Geometry check sheet. Reference: the model listing, model coordinates, mm. Face numbers are marked on the shaded views. A direction names the side the tool comes from. Give positions to 0.01 mm unless a question says otherwise; leave off trailing zeros. Write each loop counter-clockwise with the first axis right and the second up, starting at its lowest first coordinate (ties: lowest second). Pieces come first, ordered by that corner, then holes. Notation, with made-up numbers: (62, 85.25) - (118, 85.25) arc R34 ccw to (118, 120.25) - close; hole circle Ø11 at (65.25, 77). An arc over 180 degrees is marked (long way). One line per question, with ' | ' between items. Start each with the question number.
Q1. Release check for a two-part mould opening along Z. For the marked faces 1, 2 and 3 record: +Z half, -Z half, draft (parallel to the pull), parting line (faces both ways), or undercut.
Q2. Section check B-B on z = 18. Record the boundary of the cut face in (x, y) (3 decimals), and give its area (3 significant figures).
Q3. Section check A-A on x = -17. Record the boundary of the cut face in (y, z).
Q4. Set-up check for the marked faces 4 and 5: record each of +Z, -Z, +X, -X, +Y, -Y from which the full face is reachable in a straight line by a thin tool's end or side.
Q5. Section check C-C on x = -27.5. Record the boundary of the cut face in (y, z).
Q6. Section check D-D on z = 45. Record the boundary of the cut face in (x, y) (3 decimals), and give its area (3 significant figures).
Q7. Gauge pin test, flat ends, axial feed: P1, Ø1.5, axis at x = 8.5, z = 103.5, coming from the +Y side; P2, Ø6, axis at x = 17, y = 7.5, coming from the +Z side; P3, Ø4, axis at x = 6, z = 46, coming from the +Y side; P4, Ø8, axis at x = 4, z = 28, coming from the +Y side. Record the tip position at first contact, or that the pin passes through.
Q8. Thickness scan on L1, parallel to Y at x = -17, z = 104.05; L2, parallel to Z at x = 15, y = -4; L3, parallel to Y at x = 0.5, z = 99. Record the ranges inside material, lowest first. Write a range as [from, to].
Autodesk Fusion 360 part; units mm, degrees
sketch "Sketch1" plane through (0, 0, 0) normal (0, 0, 1) x (1, 0, 0)
  circle A0 centre (0, 0) radius 7
  circle A1 centre (0, 0) radius 12.5
  dimension "d1" = 25
  dimension "d2" = 14
extrude "Extrude1" add sketch "Sketch1" along normal blind 15 contours A0 | A1
sketch "Sketch2" plane through (0, 0, 15) normal (0, 0, 1) x (1, 0, 0)
  circle A0 centre (0, 0) radius 12.5
  circle A1 centre (0, 0) radius 6.375
  dimension "d5" = 12.75
loft "Loft1" cut profiles "Sketch1", "Sketch2" section 1 contours A0 section 2 contours A1
extrude "Extrude2" add 1 faces at (10.4118, -0.621, 15) along direction (0, 0, 1) blind 92
sketch "Sketch17" plane through (0, 0, 107) normal (0, 0, 1) x (1, 0, 0)
  circle A0 centre (-17, -7.5) radius 2.25
  circle A1 centre (17, -7.5) radius 2.25
  circle A2 centre (0, 0) radius 6.375
  circle A3 centre (0, 0) radius 12.5
  line L0 (-22.5, 13) -> (22.5, 13)
  line L1 (22.5, 13) -> (22.5, -13)
  line L2 (22.5, -13) -> (-22.5, -13)
  line L3 (-22.5, -13) -> (-22.5, 13)
  line L4 (0, 0) -> (-22.5, 0) construction
  line L5 (0, 0) -> (22.5, 0) construction
  circle A4 centre (-17, 7.5) radius 2.25
  circle A5 centre (17, 7.5) radius 2.25
  point P0 (-12.5, 0)
  point P1 (12.5, 0)
  dimension "d112" = 4.5
  dimension "d113" = 4.5
  dimension "d147" = 10
  dimension "d148" = 10
  dimension "d149" = 7.5
  dimension "d150" = 13
  dimension "d151" = 17
  dimension "d152" = 17
  dimension "d153" = 7.5
  dimension "d154" = 17
  dimension "d155" = 7.5
  dimension "d156" = 4.5
  dimension "d157" = 4.5
  dimension "d158" = 17
  dimension "d159" = 7.5
extrude "Extrude15" add sketch "Sketch17" against normal blind 5 contours A3 | L0 L1 L2 L3
sketch "Sketch18" plane through (0, 0, 0) normal (0, 0, -1) x (-1, 0, 0)
  circle A0 centre (-17, -7.5) radius 2.25
  circle A1 centre (17, -7.5) radius 2.25
  line L0 (-34.9564, 15) -> (34.9564, 15)
  line L1 (34.9564, 15) -> (34.9564, -15)
  line L2 (34.9564, -15) -> (-34.9564, -15)
  line L3 (-34.9564, -15) -> (-34.9564, 15)
  circle A2 centre (-27.4564, -7.5) radius 2.25
  circle A3 centre (0, 0) radius 7
  circle A4 centre (0, 0) radius 12.5
  line L4 (-22.5, -13) -> (22.5, -13)
  line L5 (22.5, -13) -> (22.5, 13)
  line L6 (22.5, 13) -> (-22.5, 13)
  line L7 (-22.5, 13) -> (-22.5, -13)
  circle A5 centre (0, 0) radius 12.5
  circle A6 centre (-17, 7.5) radius 2.25
  circle A7 centre (17, 7.5) radius 2.25
  circle A8 centre (-27.4564, 7.5) radius 2.25
  circle A9 centre (27.4564, 7.5) radius 2.25
  point P0 (0, -15)
  dimension "d122" = 4.5
  dimension "d124" = 7.5
  dimension "d125" = 7.5
  dimension "d160" = 34.9564
  dimension "d161" = 15
  dimension "d162" = 34.9564
  dimension "d163" = 15
  dimension "d164" = 7.5
  dimension "d165" = 7.5
  dimension "d166" = 4.5
  dimension "d167" = 7.5
  dimension "d168" = 7.5
  dimension "d169" = 4.5
extrude "Extrude16" add sketch "Sketch18" against normal blind 3 contours A0 | A1 | L0 L1 L2 L3 | L4 L5 L6 L7 | A6 | A7
ref_plane "WorkPlane5" through (0, -7, 0) normal (0, 1, 0) x (0, 0, 1)
sketch "Sketch19" plane through (0, -7, 0) normal (0, 1, 0) x (1, 0, 0)
  line L0 (6.375, -15) -> (-6.375, -15)
  line L1 (0, -15) -> (0, -107) construction
  circle A0 centre (0, -18) radius 1.7
  circle A1 centre (0, -18) radius 2.7
  line L2 (6.375, -107) -> (-6.375, -107)
  dimension "d131" = 3.4
  dimension "d132" = 5.4
  dimension "d139" = 3
extrude "Extrude17" add sketch "Sketch19" against normal blind 8
extrude "Extrude18" cut sketch "Sketch19" along normal blind 2 and the other way blind 8 contours A0
ref_plane "WorkPlane7" through (0, 7, 0) normal (0, 1, 0) x (0, 0, 1)
sketch "Sketch22" plane through (0, 7, 0) normal (0, 1, 0) x (1, 0, 0)
  circle A0 centre (0, -18) radius 1.7
  circle A1 centre (0, -18) radius 2.7
  point P0 (0, -18)
  dimension "d171" = 3.4
  dimension "d172" = 5.4
extrude "Extrude21" add sketch "Sketch22" along normal blind 8
extrude "Extrude22" cut sketch "Sketch22" along normal blind 8 and the other way blind 2 contours A0
sketch "Sketch23" plane through (0, 0, 0) normal (0, 0, -1) x (-1, 0, 0)
  line L0 (-34.9564, -15) -> (34.9564, -15)
  line L1 (34.9564, -15) -> (34.9564, 15)
  line L2 (34.9564, 15) -> (-34.9564, 15)
  line L3 (-34.9564, 15) -> (-34.9564, -15)
  circle A0 centre (-27.4564, 7.5) radius 2.25
  circle A1 centre (-27.4564, -7.5) radius 2.25
  circle A2 centre (27.4564, 7.5) radius 2.25
  circle A3 centre (0, 0) radius 7
  line L4 (34.9564, -15) -> (30.1724, -15)
  line L5 (34.9564, -9.125) -> (34.9564, -15)
  arc A4 (34.9564, -9.125) -> (30.1724, -15) centre (36.8966, -15.5902) ccw
  dimension "d181" = 4.784
  dimension "d182" = 5.875
  dimension "d183" = 6.75
extrude "Extrude23" cut sketch "Sketch23" against normal up to surface (3 mm away) contours L0 L1 L4 L5 A4
equation "d113 = d112"
equation "d116 = d110 / 2"
equation "d125 = d124"
equation "d130 = -d2 / 2"
equation "d132 = d131 + 2 mm"
equation "d148 = d147"
equation "d152 = d151"
equation "d153 = d149"
equation "d154 = d151"
equation "d155 = d149"
equation "d156 = d112"
equation "d157 = d112"
equation "d158 = d151"
equation "d159 = d149"
equation "d162 = d160"
equation "d163 = d161"
equation "d164 = d124"
equation "d165 = d124"
equation "d166 = d122"
equation "d167 = d124"
equation "d168 = d124"
equation "d169 = d122"
equation "d170 = ( d2 / 2 mm ) * 1 mm"
equation "d172 = d171 + 2 mm"
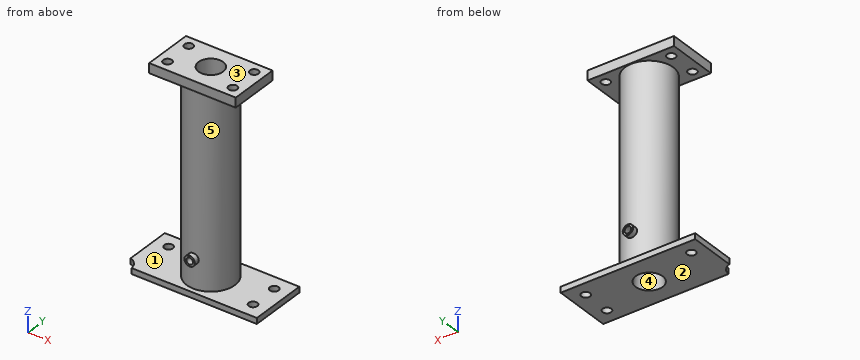
Working result:
1) face 1: undercut | face 2: -Z half | face 3: +Z half
2) outline: (-2.7, -15) - (-1.7, -15) - (-1.7, -6.144) arc R6.375 cw to (-1.7, 6.144) - (-1.7, 15) - (-2.7, 15) - (-2.7, 12.205) arc R12.5 ccw to (-2.7, -12.205) - close; (1.7, -15) - (2.7, -15) - (2.7, -12.205) arc R12.5 ccw to (2.7, 12.205) - (2.7, 15) - (1.7, 15) - (1.7, 6.144) arc R6.375 cw to (1.7, -6.144) - close | area: 332 mm2
3) outline: (-15, 0) - (15, 0) - (15, 3) - (-15, 3) - close; (-13, 102) - (-9.75, 102) - (-9.75, 107) - (-13, 107) - close; (-5.25, 102) - (5.25, 102) - (5.25, 107) - (-5.25, 107) - close; (9.75, 102) - (13, 102) - (13, 107) - (9.75, 107) - close
4) face 4: -Z | face 5: none
5) outline: (-15, 0) - (5.25, 0) - (5.25, 3) - (-15, 3) - close; (9.75, 0) - (15, 0) - (15, 3) - (9.75, 3) - close
6) outline: circle Ø25 at (0, 0); hole circle Ø12.75 at (0, 0) | area: 363 mm2
7) P1: stops at y = 13 | P2: stops at z = 107 | P3: stops at y = 11.84 | P4: stops at y = 12.5
8) L1: y = [-13, -9.75], [-5.25, 5.25], [9.75, 13] | L2: z = [0, 3], [102, 107] | L3: y = [-12.49, -6.36], [6.36, 12.49]
